```python
from build123d import *

# Parameters (mm, degrees)
BOSS_EXTRUDE1_DEPTH     = 53.975
CUT_EXTRUDE1_DEPTH      = 55.780368286
CUT_EXTRUDE1_DEPTH_BACK = 55.780368286
SKETCH2_R               = 2.4892


with BuildPart() as part:
    # Sketch1 → Boss-Extrude1 (new body)
    with BuildSketch(Plane.XY):
        with BuildLine():
            ThreePointArc((6.35, 2.634980936), (5.953924622, 3.437499983), (5.456960429, 4.181770846))
            Line((5.456960429, 4.181770846), (0.893039571, 6.816751782))
            ThreePointArc((0.893039571, 6.816751782), (0, 6.874999966), (-0.893039571, 6.816751782))
            Line((-0.893039571, 6.816751782), (-5.456960429, 4.181770846))
            ThreePointArc((-5.456960429, 4.181770846), (-5.953924622, 3.437499983), (-6.35, 2.634980936))
            Line((-6.35, 2.634980936), (-6.35, -2.634980936))
            ThreePointArc((-6.35, -2.634980936), (-5.953924622, -3.437499983), (-5.456960429, -4.181770846))
            Line((-5.456960429, -4.181770846), (-0.893039571, -6.816751782))
            ThreePointArc((-0.893039571, -6.816751782), (0, -6.874999966), (0.893039571, -6.816751782))
            Line((0.893039571, -6.816751782), (5.456960429, -4.181770846))
            ThreePointArc((5.456960429, -4.181770846), (5.953924622, -3.437499983), (6.35, -2.634980936))
            Line((6.35, -2.634980936), (6.35, 2.634980936))
        make_face()
    extrude(amount=BOSS_EXTRUDE1_DEPTH)

    # Sketch2 → Cut-Extrude1 (cut, two sides: drawn at the far end of the back side and taken through both)
    with BuildSketch(Plane(origin=(0, 0, 0), x_dir=(-1, 0, 0), z_dir=(0, 0, -1)).offset(-CUT_EXTRUDE1_DEPTH_BACK)):
        Circle(SKETCH2_R)
    extrude(amount=CUT_EXTRUDE1_DEPTH + CUT_EXTRUDE1_DEPTH_BACK, mode=Mode.SUBTRACT)


solid = part.part
```
Geometry: final body of the model. Coordinates: model frame, mm. Coordinates: 2 decimals unless noted, no trailing zeros. Order: outer loops, then holes, each group sorted by start corner. A loop starts at its lowest first (then second) coordinate and runs counter-clockwise, first axis right, second up.
Item 1: Section query B-B (y = -1.75). Output: boundary loops of the cut face in (x, z) (3 decimals), then the cut area to 3 significant figures.
Answer:
outline: (-6.35, 0) - (-1.77, 0) - (-1.77, 53.975) - (-6.35, 53.975) - close; (1.77, 0) - (6.35, 0) - (6.35, 53.975) - (1.77, 53.975) - close
area: 494 mm2
Item 2: Section query D-D (x = -3). Output: boundary loops of the cut face in (y, z) (3 decimals).
Answer:
outline: (-5.6, 0) - (5.6, 0) - (5.6, 53.975) - (-5.6, 53.975) - close
Item 3: Material intervals for line 1 along X through (y, z) = (0, 34); line 2 along Y through (x, z) = (0, 38) (3 decimals); line 3 along Y through (x, z) = (-3.25, 30), sorted ascending.
Answer:
line 1: x = -6.35 to -2.49, 2.49 to 6.35
line 2: y = -6.875 to -2.489, 2.489 to 6.875
line 3: y = -5.46 to 5.46
Item 4: Section query C-C (z = 40.5). Output: boundary loops of the cut face in (x, y) (3 decimals), then the cut area to 3 significant figures.
Answer:
outline: (-6.35, -2.635) arc R6.875 ccw to (-5.457, -4.182) - (-0.893, -6.817) arc R6.875 ccw to (0.893, -6.817) - (5.457, -4.182) arc R6.875 ccw to (6.35, -2.635) - (6.35, 2.635) arc R6.875 ccw to (5.457, 4.182) - (0.893, 6.817) arc R6.875 ccw to (-0.893, 6.817) - (-5.457, 4.182) arc R6.875 ccw to (-6.35, 2.635) - close; hole circle Ø4.978 at (0, 0)
area: 118 mm2
Item 5: Draft query along X for faces 1 (the face through (-2.374, 0.748, 27.365)), 2 (the face through (-0.013, -6.875, 26.61)), 3 (the face through (-3.14, 5.52, 26.61)). Return one class per face: released by +X, released by -X, zero draft, split by the parting line, or undercut.
Answer:
face 1: undercut
face 2: split by the parting line
face 3: released by -X
Item 6: Section query A-A (x = 0). Output: boundary loops of the cut face in (y, z) (3 decimals), then the cut area to 3 significant figures.
Answer:
outline: (-6.875, 0) - (-2.489, 0) - (-2.489, 53.975) - (-6.875, 53.975) - close; (2.489, 0) - (6.875, 0) - (6.875, 53.975) - (2.489, 53.975) - close
area: 473 mm2
Item 7: Contact query for flat-ended pins moving along their axis: P1, Ø2, axis at x = -3, z = 39, coming from the +Y side; P2, Ø3, axis at y = -5, z = 11, coming from the -X side. Output: stop coordinate, or through.
Answer:
P1: stops at y = 6.18
P2: stops at x = -5.92
